Part model, mm, in its own coordinate system. Coordinates: 2 decimals unless noted, no trailing zeros. Write each loop counter-clockwise with the first axis right and the second up, starting at its lowest first coordinate (ties: lowest second). Pieces come first, ordered by that corner, then holes. Notation, with made-up numbers: (83.5, -19) - (129.5, -19) arc R33 ccw to (129.5, 9) - close; hole circle Ø2 at (-13.5, 37.5). An arc over 180 degrees is marked (long way). Use one line per item in the form item = value. Start each with the question number.
Autodesk Inventor part; units mm, degrees
ref_plane "XZ Plane" through (0, 0, 0) normal (0, 1, 0) x (-1, 0, 0)
ref_plane "XY Plane" through (0, 0, 0) normal (0, 0, 1) x (1, 0, 0)
sketch "Skizze1" plane through (0, 0, 0) normal (0, 1, 0) x (-1, 0, 0)
  line L0 (4, 0) -> (4, -7.5)
  line L1 (4, -7.5) -> (3, -7.5)
  line L2 (7.5, -15) -> (7.5, 0)
  line L3 (7.5, 0) -> (4, 0)
  line L4 (0, 3.7992) -> (0, -25.1489)
  line L5 (7.5, -15) -> (3, -15)
  line L6 (3, -15) -> (3, -10)
  line L7 (3, -10) -> (3, -10)
  line L8 (3, -10) -> (3, -7.5)
  point P0 (0, 0)
  dimension "d6" = 4
  dimension "d9" = 4.5
  dimension "d10" = 5
  dimension "d15" = 6
  dimension "d16" = 15
  dimension "d17" = 7.5
  dimension "d18" = 15
revolve "Umdrehung1" add sketch "Skizze1" angle 360 about axis through (0, 0, 3.7992) along (0, 0, -1)
thread "Gewinde1"
thread "Gewinde2"
ref_plane "Arbeitsebene1" through (7.5, 0, 0) normal (1, 0, 0) x (0, 1, 0)
sketch "Skizze3" plane through (7.5, 0, 0) normal (1, 0, 0) x (0, 1, 0)
  line L0 (-4, -7.5) -> (4, -7.5)
  line L1 (-7.5, -15) -> (7.5, -15)
  line L2 (0, 0) -> (0, -15)
  line L3 (-3, -15) -> (3, -15)
  point P0 (0, -11.25)
  dimension "d20" = 3.75
hole "Bohrung1" at (7.5, 0, -11.25) direction (-1, 0, 0) diameter 2.459 end up to surface
properties part number "Glasdeckel"
Q1. Slice it at B-B (x = 0). List the corners of the cut face in (y, z), plus the area to 3 significant figures.
Q2. Pin check, flat tips, straight feed: P1, Ø7, axis at x = 0, y = 0, coming from the +Z side; P2, Ø2, axis at x = -3, z = -10, coming from the -Y side; P3, Ø2, axis at y = -3.5, z = -10.5, coming from the +X side. Stop position of each tip, or through.
Q3. Slice it at C-C (y = -2.75). List the corners of the cut face in (x, z), plus the area to 3 significant figures.
Q4. Mould opens along Z. For faces 1 (the flat face through (0.1, -3.2, -15)), 2 (the flat face through (-1, 3, -7.5)), 3 (the cylindrical face through (0.867, -3.905, -3.802)), 4 (the cylindrical face through (5.1, 1.1, -11.8)) say: released by +Z, released by -Z, zero draft, split by the parting line, or undercut.
Q5. Drill centre lines: probe 1 along Y at (x, z) = (0, -12); probe 2 along Y at (x, z) = (0, -3.75); probe 3 along X at (y, z) = (2.25, -4.25). Where is each one in solid material? Low to high.
Q6. Slice it at D-D (x = 5). List the corners of the cut face in (y, z), plus the area to 3 significant figures.
Q7. Slice it at A-A (y = 0). List the corners of the cut face in (x, z).
Solution:
q1.outline = (-7.5, -15) - (-3, -15) - (-3, -7.5) - (-4, -7.5) - (-4, 0) - (-7.5, 0) - close; (3, -15) - (7.5, -15) - (7.5, 0) - (4, 0) - (4, -7.5) - (3, -7.5) - close
q1.area = 120 mm2
q2.P1 = -7.5
q2.P2 = -7.23
q2.P3 = 7.07
q3.outline = (-6.98, -15) - (-1.2, -15) - (-1.2, -7.5) - (-2.9, -7.5) - (-2.9, 0) - (-6.98, 0) - close; (1.2, -15) - (6.98, -15) - (6.98, 0) - (2.9, 0) - (2.9, -7.5) - (1.2, -7.5) - close
q3.area = 148 mm2
q4.face_1 = released by -Z
q4.face_2 = released by +Z
q4.face_3 = zero draft
q4.face_4 = undercut
q5.probe_1 = -7.5 to -3, 3 to 7.5
q5.probe_2 = -7.5 to -4, 4 to 7.5
q5.probe_3 = -7.15 to -3.31, 3.31 to 7.15
q6.outline = (-5.59, -15) - (5.59, -15) - (5.59, 0) - (-5.59, 0) - close; hole circle Ø2.46 at (0, -11.25)
q6.area = 163 mm2
q7.outline = (-7.5, -15) - (-3, -15) - (-3, -7.5) - (-4, -7.5) - (-4, 0) - (-7.5, 0) - close; (3, -15) - (7.5, -15) - (7.5, -12.48) - (3, -12.48) - close; (3, -10.02) - (7.5, -10.02) - (7.5, 0) - (4, 0) - (4, -7.5) - (3, -7.5) - close
